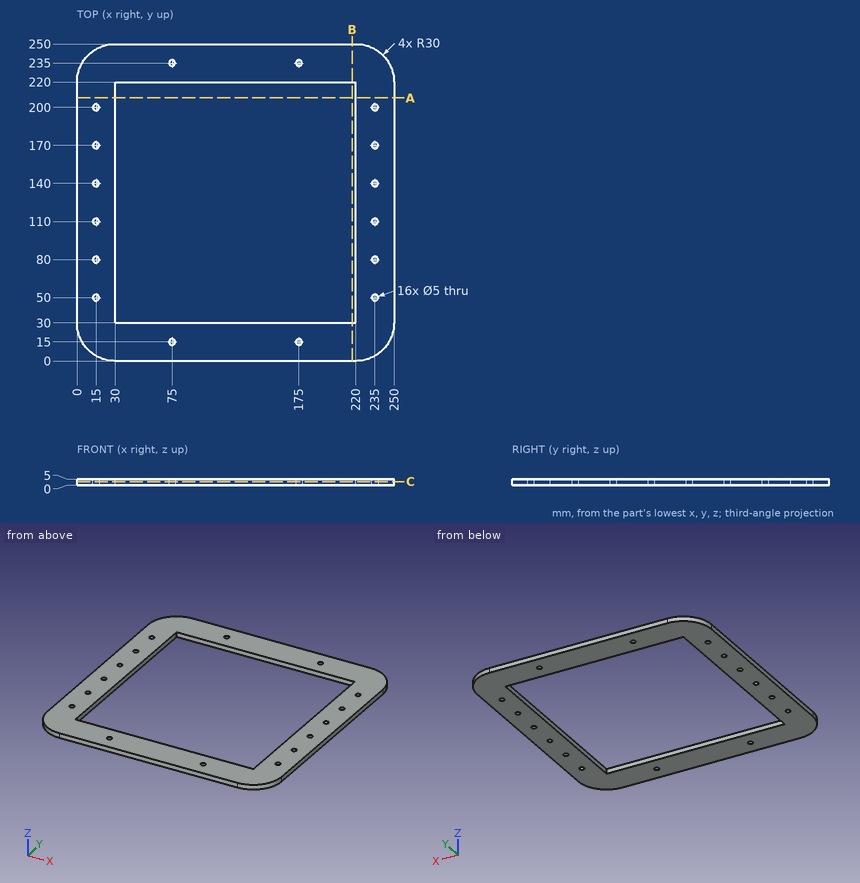
Verification items for this drawing (mm, ordinates from the low corner). Round coordinates to 2 decimals unless told otherwise and drop trailing zeros. Write each loop counter-clockwise with the first axis right and the second up, starting at its lowest first coordinate (ties: lowest second). Pieces come first, ordered by that corner, then holes. Notation, with made-up numbers: (16, 57) - (56, 57) arc R12 cw to (56, 74) - close; hole circle Ø9 at (-30, 36.5). An arc over 180 degrees is marked (long way). Answer as a JSON object with one key per item and string values. Group by question number.
Q1. Section check C-C, the plane z = 2.85. Give the number of separate pieces and of enclosed holes in the cut face, plus the area to 3 significant figures.
Q2. Section check A-A, the plane y = 207.5. Enter the section's corners in (x, z).
Q3. Go/stop test with a flat-tipped pin: pin 1 Ø4 at (x, y) = (15, 140) entering from -Z. Record where the tip stops, or that it passes through.
Q4. Thickness scan on line 1 (X direction, y = 200, z = 2.4); line 2 (X direction, y = 106, z = 3.1). Record the ranges inside material, lowest first.
Found:
{
 "1": {"separate pieces": "1", "enclosed holes": "17", "area": "25,300 mm^2"},
 "2": {"outline": "(0, 0) - (30, 0) - (30, 5) - (0, 5) - close; (220, 0) - (250, 0) - (250, 5) - (220, 5) - close"},
 "3": {"pin 1": "passes through"},
 "4": {"line 1": "x = 0 to 12.5, 17.5 to 30, 220 to 232.5, 237.5 to 250", "line 2": "x = 0 to 30, 220 to 250"}
}
